Source: CAD feature listing. Evaluate the final solid. Frame: model axes, mm. A direction names the side the tool comes from. Give positions to 0.01 mm unless a question says otherwise; leave off trailing zeros. Loops run counter-clockwise (first coordinate to the right, second up) from the corner with the lowest first, then second, coordinate; pieces in that order, holes last.
from build123d import *

# Parameters (mm, degrees)
SKETCH2_W           = 110
SKETCH2_H           = 118
BOSS_EXTRUDE1_DEPTH = 4
SKETCH3_W           = 10
SKETCH3_H           = 62
BOSS_EXTRUDE2_DEPTH = 16
CUT_EXTRUDE8_DEPTH  = 163.55460621
SKETCH12_W          = 6
SKETCH12_H          = 16
BOSS_EXTRUDE3_DEPTH = 16
SKETCH14_R          = 4
CUT_EXTRUDE9_DEPTH  = 156.961533719
CUT_EXTRUDE10_DEPTH = 3.5
SKETCH24_R          = 3
CUT_EXTRUDE15_DEPTH = 8
SPLIT2_OUTLINE_W    = 16
SPLIT2_OUTLINE_H    = 62
SPLIT2_DEPTH        = 110
SPLIT3_START        = 10
SPLIT3_OUTLINE_W    = 16
SPLIT3_OUTLINE_H    = 16
SPLIT3_OUTLINE_R    = 4
SPLIT3_DEPTH        = 90
SKETCH25_W          = 10
SKETCH25_H          = 62
SKETCH25_W_2        = 6
SKETCH25_H_2        = 16
CUT_EXTRUDE16_DEPTH = 10
SKETCH27_R          = 3.395097118
SKETCH27_R_2        = 3.39905673
BOSS_EXTRUDE4_DEPTH = 4
BOSS_EXTRUDE5_DEPTH = 2
CUT_EXTRUDE18_START = -6
SKETCH29_R          = 3
SKETCH29_W          = 6
SKETCH29_H          = 16
CUT_EXTRUDE18_DEPTH = 6
SKETCH30_W          = 4
SKETCH30_H          = 56
CUT_EXTRUDE19_DEPTH = 10


# Read off the part's stored shape, not the designer's step: Split2, Split3
with BuildPart() as part:
    # Sketch2 → Boss-Extrude1 (new body)
    with BuildSketch(Plane(origin=(0, 0, 0), x_dir=(1, 0, 0), z_dir=(0, 1, 0))):
        with Locations((55, 59)):
            Rectangle(SKETCH2_W, SKETCH2_H)
    extrude(amount=BOSS_EXTRUDE1_DEPTH)

    # Sketch3 → Boss-Extrude2 (add)
    with BuildSketch(Plane(origin=(0, 4, 0), x_dir=(1, 0, 0), z_dir=(0, 1, 0))):
        with Locations((5, 87)):
            Rectangle(SKETCH3_W, SKETCH3_H)
        with Locations((105, 87)):
            Rectangle(SKETCH3_W, SKETCH3_H)
    extrude(amount=BOSS_EXTRUDE2_DEPTH)

    # Sketch11 → Cut-Extrude8 (cut, through all)
    with BuildSketch(Plane.ZY):
        with BuildLine():
            Line((-111, 17.105440781), (-63, 17.105440781))
            ThreePointArc((-63, 17.105440781), (-59, 13.105440781), (-63, 9.105440781))
            Line((-63, 9.105440781), (-111, 9.105440781))
            ThreePointArc((-111, 9.105440781), (-115, 13.105440781), (-111, 17.105440781))
        make_face()
    extrude(amount=-CUT_EXTRUDE8_DEPTH, mode=Mode.SUBTRACT)

    # Sketch12 → Boss-Extrude3 (add)
    with BuildSketch(Plane(origin=(0, 4, 0), x_dir=(1, 0, 0), z_dir=(0, 1, 0))):
        with Locations((13, 23)):
            Rectangle(SKETCH12_W, SKETCH12_H)
        with Locations((97, 23)):
            Rectangle(SKETCH12_W, SKETCH12_H)
        with Locations((84.65, 23)):
            Rectangle(SKETCH12_W, SKETCH12_H)
        with Locations((25.35, 23)):
            Rectangle(SKETCH12_W, SKETCH12_H)
    extrude(amount=BOSS_EXTRUDE3_DEPTH)

    # Sketch14 → Cut-Extrude9 (cut, through all)
    with BuildSketch(Plane.ZY.offset(-10)):
        with Locations((-23, 14)):
            Circle(SKETCH14_R)
    extrude(amount=-CUT_EXTRUDE9_DEPTH, mode=Mode.SUBTRACT)

    # Sketch16 → Cut-Extrude10 (cut)
    with BuildSketch(Plane(origin=(10, 0, 0), x_dir=(0, 0, -1), z_dir=(1, 0, 0))):
        Polygon((74.219115806, 19.439463765), (74.219115806, 18.227285811), (62.862799814, 18.227285811), (62.862799814, 19.672541564), (62.862799814, 20.227285811), (74.219115806, 20.227285811), align=None)
    cut_extrude10 = extrude(amount=-CUT_EXTRUDE10_DEPTH, mode=Mode.SUBTRACT)

    # Mirror1: Cut-Extrude10 across plane
    add(cut_extrude10.mirror(Plane(origin=(55, 0, 0), x_dir=(0, 0, 1), z_dir=(1, 0, 0))), mode=Mode.SUBTRACT)

    # Sketch24 → Cut-Extrude15 (cut)
    with BuildSketch(Plane.XZ):
        with Locations(Location((65.746814509, -111.493629018, 0), (0, 0, 270))):
            Circle(SKETCH24_R)
        with Locations(Location((43.746814509, -111.493629018, 0), (0, 0, 270))):
            Circle(SKETCH24_R)
        with Locations(Location((65.746814509, -15.493629018, 0), (0, 0, 270))):
            Circle(SKETCH24_R)
        with Locations(Location((43.746814509, -15.493629018, 0), (0, 0, 270))):
            Circle(SKETCH24_R)
        with Locations(Location((102.746814509, -52.493629018, 0), (0, 0, 270))):
            Circle(SKETCH24_R)
        with Locations(Location((6.746814509, -52.493629018, 0), (0, 0, 270))):
            Circle(SKETCH24_R)
    extrude(amount=-CUT_EXTRUDE15_DEPTH, mode=Mode.SUBTRACT)

    # Split2 outline → Split2 (cut)
    with BuildSketch(Plane.YZ):
        with Locations((12, -87)):
            Rectangle(SPLIT2_OUTLINE_W, SPLIT2_OUTLINE_H)
        with BuildLine():
            Line((9.105440781, -111), (9.105440781, -63))
            ThreePointArc((9.105440781, -63), (13.105440781, -59), (17.105440781, -63))
            Line((17.105440781, -63), (17.105440781, -111))
            ThreePointArc((17.105440781, -111), (13.105440781, -115), (9.105440781, -111))
        make_face(mode=Mode.SUBTRACT)
    extrude(amount=SPLIT2_DEPTH, mode=Mode.SUBTRACT)

    # Split3 outline → Split3 (cut)
    with BuildSketch(Plane.YZ.offset(SPLIT3_START)):
        with Locations((12, -23)):
            Rectangle(SPLIT3_OUTLINE_W, SPLIT3_OUTLINE_H)
        with Locations((14, -23)):
            Circle(SPLIT3_OUTLINE_R, mode=Mode.SUBTRACT)
    extrude(amount=SPLIT3_DEPTH, mode=Mode.SUBTRACT)

    # Sketch25 → Cut-Extrude16 (cut)
    with BuildSketch(Plane(origin=(0, 4, 0), x_dir=(1, 0, 0), z_dir=(0, 1, 0))):
        with Locations((5, 87)):
            Rectangle(SKETCH25_W, SKETCH25_H)
        with Locations((13, 23)):
            Rectangle(SKETCH25_W_2, SKETCH25_H_2)
        with Locations((25.35, 23)):
            Rectangle(SKETCH25_W_2, SKETCH25_H_2)
        with Locations((84.65, 23)):
            Rectangle(SKETCH25_W_2, SKETCH25_H_2)
        with Locations((97, 23)):
            Rectangle(SKETCH25_W_2, SKETCH25_H_2)
        with Locations((105, 87)):
            Rectangle(SKETCH25_W, SKETCH25_H)
    extrude(amount=-CUT_EXTRUDE16_DEPTH, mode=Mode.SUBTRACT)

    # Sketch27 → Boss-Extrude4 (add)
    with BuildSketch(Plane(origin=(0, 4, 0), x_dir=(1, 0, 0), z_dir=(0, 1, 0))):
        with Locations((6.746814509, 52.493629018)):
            Circle(SKETCH27_R)
        with Locations((102.746814509, 52.493629018)):
            Circle(SKETCH27_R_2)
    extrude(amount=-BOSS_EXTRUDE4_DEPTH)

    # Sketch28 → Boss-Extrude5 (add)
    with BuildSketch(Plane.XZ):
        Polygon((100, -56), (110, -56), (110, 0), (0, 0), (0, -56), (10, -56), (10, -118), (100, -118), align=None)
    extrude(amount=BOSS_EXTRUDE5_DEPTH)

    # Sketch29 → Cut-Extrude18 (cut)
    with BuildSketch(Plane(origin=(0, 4, 0), x_dir=(1, 0, 0), z_dir=(0, 1, 0)).offset(CUT_EXTRUDE18_START)):
        with Locations(Location((43.746814509, 111.493629018, 0), (0, 0, 90))):
            Circle(SKETCH29_R)
        with Locations(Location((65.746814509, 111.493629018, 0), (0, 0, 90))):
            Circle(SKETCH29_R)
        with Locations(Location((43.746814509, 15.493629018, 0), (0, 0, 90))):
            Circle(SKETCH29_R)
        with Locations(Location((65.746814509, 15.493629018, 0), (0, 0, 90))):
            Circle(SKETCH29_R)
        with Locations((25.35, 23)):
            Rectangle(SKETCH29_W, SKETCH29_H)
        with Locations((13, 23)):
            Rectangle(SKETCH29_W, SKETCH29_H)
        with Locations((84.65, 23)):
            Rectangle(SKETCH29_W, SKETCH29_H)
        with Locations((97, 23)):
            Rectangle(SKETCH29_W, SKETCH29_H)
    extrude(amount=CUT_EXTRUDE18_DEPTH, mode=Mode.SUBTRACT)

    # Sketch30 → Cut-Extrude19 (cut)
    with BuildSketch(Plane(origin=(0, 4, 0), x_dir=(1, 0, 0), z_dir=(0, 1, 0))):
        with Locations((2, 28)):
            Rectangle(SKETCH30_W, SKETCH30_H)
        with Locations((108, 28)):
            Rectangle(SKETCH30_W, SKETCH30_H)
    extrude(amount=-CUT_EXTRUDE19_DEPTH, mode=Mode.SUBTRACT)


solid = part.part
1) Ray query, probe 1 along X at (y, z) = (0.45, -26); probe 2 along Z at (x, y) = (26, 1.7); probe 3 along X at (y, z) = (-1.55, -110). Return the intervals inside material, ascending.
Checks:
probe 1: x = 4 to 10, 16 to 22.35, 28.35 to 81.65, 87.65 to 94, 100 to 106
probe 2: z = -118 to -31, -15 to 0
probe 3: x = 10 to 41.15, 46.35 to 63.15, 68.35 to 100
2) Cut plane A-A (z = -28). Return loops of the section in (x, y), and give its area (3 significant figures).
Checks:
outline: (4, -2) - (10, -2) - (10, 4) - (4, 4) - close; (16, -2) - (22.35, -2) - (22.35, 4) - (16, 4) - close; (28.35, -2) - (81.65, -2) - (81.65, 4) - (28.35, 4) - close; (87.65, -2) - (94, -2) - (94, 4) - (87.65, 4) - close; (100, -2) - (106, -2) - (106, 4) - (100, 4) - close
area: 468 mm2
3) Cut plane C-C (z = -82.5). Return loops of the section in (x, y), and give its area (3 significant figures).
Checks:
outline: (10, -2) - (100, -2) - (100, 4) - (10, 4) - close
area: 540 mm2
4) Cut plane B-B (y = 1.8). State how many separate pieces and enclosed holes the cut face has, and give its area (3 significant figures).
Checks:
separate pieces: 1
enclosed holes: 8
area: 10,800 mm2
5) Pull-direction query (X, two-part tool) for faces 4 (the flat face through (100, 1, -23)), 5 (the flat face through (106, 1, -28)), 6 (the flat face through (103, 1, -56)); classes: released by +X, released by -X, zero draft, split by the parting line, or undercut.
Checks:
face 4: undercut
face 5: released by +X
face 6: zero draft
6) Reachability of faces 1 (the flat face through (7, 1, -56)), 2 (the flat face through (28.35, 1, -23)), 3 (the flat face through (54, 4, -60)) from +Z, -Z, +X, -X, +Y, -Y: full face, straight path, thin tool, end or side. Return the list, or none.
Checks:
face 1: -Z, -X, +Y, -Y
face 2: +Y, -Y
face 3: +Z, -Z, +X, -X, +Y
7) Contact query for a flat-ended pin moving along its axis: P1, Ø3, axis at y = 2, z = -83.5, coming from the +X side. Output: stop coordinate, or through.
Checks:
P1: stops at x = 100
